CAD build for the part. Positions are in the model's coordinates, mm. Face numbers are marked on the shaded views. A direction names the side the tool comes from. Coordinates: 2 decimals unless noted, no trailing zeros. Loops run counter-clockwise (first coordinate to the right, second up) from the corner with the lowest first, then second, coordinate; pieces in that order, holes last. Notation, with made-up numbers: (-25, 1.25) - (30, 1.25) arc R21 ccw to (30, 22.25) - close; hole circle Ø3 at (-36.75, 60). An arc over 180 degrees is marked (long way). Put each result on its own line as item: value.
Autodesk Inventor part; units mm, degrees
ref_plane "YZ Plane" through (0, 0, 0) normal (1, 0, 0) x (0, 1, 0)
ref_plane "XZ Plane" through (0, 0, 0) normal (0, 1, 0) x (-1, 0, 0)
ref_plane "XY Plane" through (0, 0, 0) normal (0, 0, 1) x (1, 0, 0)
sketch "Sketch1" plane through (0, 0, 0) normal (0, 1, 0) x (-1, 0, 0)
  line L0 (150, 125) -> (-150, 125)
  line L1 (-150, 125) -> (-150, -125)
  line L2 (-150, -125) -> (150, -125)
  line L3 (150, -125) -> (150, 125)
  point P0 (0, 0)
  dimension "d0" = 300
  dimension "d1" = 250
  dimension "d2" = 125
  dimension "d29" = 150
extrude "Plate1" add sketch "Sketch1" along normal blind 9.5
sketch "Sketch4" plane through (0, 9.5, 0) normal (0, 1, 0) x (1, 0, 0)
  line L0 (-106, -70) -> (106, -70)
  line L1 (106, -70) -> (106, 70)
  line L2 (106, 70) -> (-106, 70)
  line L3 (-106, 70) -> (-106, -70)
  line L4 (-150, -125) -> (-150, 125)
  point P0 (0, 0)
  point P1 (-130, -106)
  point P2 (-130, 106)
  dimension "d24" = 140
  dimension "d25" = 212
  dimension "d27" = 70
  dimension "d28" = 106
hole "Hole1" at (-106, 9.5, 70) at (-106, 9.5, -70) at (106, 9.5, 70) at (106, 9.5, -70) direction (0, -1, 0) diameter 12 depth 9.5
sketch "Sketch8" plane through (-140.5, 9.5, 125) normal (-1, 0, 0) x (0, 1, 0)
  line L0 (0, -250) -> (0, 0)
  line L1 (0, 0) -> (-64.5, 0)
  line L2 (-64.5, 0) -> (-64.5, -250)
  line L3 (-64.5, -250) -> (0, -250)
edge flange "Flange5" height 64.5 angle 90 thickness 9.5 bend radius 9.5 thickness toward (-1, 0, 0) relief tear relief width 9.5 relief depth 4.75 edges at (-150, 9.5, 0) wall of the first edge with corners at (-140.5, 9.5, -125) (-140.5, 9.5, 125) (-140.5, -55, 125) (-140.5, -55, -125)
bend "Bend5"
corner "Corner5"
sketch "Sketch9" plane through (140.5, 9.5, -125) normal (1, 0, 0) x (0, -1, 0)
  line L0 (0, 250) -> (0, 0)
  line L1 (0, 0) -> (64.5, 0)
  line L2 (64.5, 0) -> (64.5, 250)
  line L3 (64.5, 250) -> (0, 250)
edge flange "Flange6" height 64.5 angle 90 thickness 9.5 bend radius 9.5 thickness toward (1, 0, 0) relief tear relief width 9.5 relief depth 4.75 edges at (150, 9.5, 0) wall of the first edge with corners at (140.5, 9.5, 125) (140.5, 9.5, -125) (140.5, -55, -125) (140.5, -55, 125)
bend "Bend6"
corner "Corner6"
sketch "Sketch10" plane through (-140.5, -45.5, -125) normal (0, -1, 0) x (-1, 0, 0)
  line L0 (0, 250) -> (0, 0)
  line L1 (0, 0) -> (54.5, 0)
  line L2 (54.5, 0) -> (54.5, 250)
  line L3 (54.5, 250) -> (0, 250)
edge flange "Flange7" height 45 angle 90 thickness 9.5 bend radius 9.5 thickness toward (0, -1, 0) relief tear relief width 9.5 relief depth 4.75 edges at (-140.5, -55, 0) wall of the first edge with corners at (-140.5, -45.5, 125) (-140.5, -45.5, -125) (-195, -45.5, -125) (-195, -45.5, 125)
bend "Bend7"
corner "Corner7"
sketch "Sketch11" plane through (140.5, -45.5, 125) normal (0, -1, 0) x (-1, 0, 0)
  line L0 (0, -250) -> (0, 0)
  line L1 (0, 0) -> (-54.5, 0)
  line L2 (-54.5, 0) -> (-54.5, -250)
  line L3 (-54.5, -250) -> (0, -250)
edge flange "Flange8" height 45 angle 90 thickness 9.5 bend radius 9.5 thickness toward (0, -1, 0) relief tear relief width 9.5 relief depth 4.75 edges at (140.5, -55, 0) wall of the first edge with corners at (140.5, -45.5, -125) (140.5, -45.5, 125) (195, -45.5, 125) (195, -45.5, -125)
bend "Bend8"
corner "Corner8"
sketch "Sketch12" plane through (-195, -45.5, 125) normal (0, 1, 0) x (1, 0, 0)
  line L0 (35.5, 250) -> (0, 250)
  line L1 (17.75, 250) -> (17.75, 0)
  line L2 (35.5, 0) -> (0, 0)
  line L3 (0, 0) -> (0, 250)
  line L4 (0, 195) -> (35.5, 195)
  line L5 (0, 55) -> (35.5, 55)
  line L6 (35.5, 250) -> (35.5, 0)
  point P0 (195, 125)
  point P1 (17.75, 195)
  point P2 (17.75, 55)
  dimension "d110" = 55
  dimension "d111" = 55
hole "Hole3" at (-177.25, -45.5, -70) at (-177.25, -45.5, 70) direction (0, -1, 0) diameter 12 depth 9.5
mirror "Mirror2" about plane through (0, 0, 0) normal (1, 0, 0) of "Hole3"
equation "\"d35\" = Thickness"
equation "\"d117\" = Thickness"
equation "\"d3\" = Thickness"
equation "\"d69\" = BendReliefWidth"
equation "\"d70\" = BendReliefDepth"
equation "\"d71\" = MinimumRemnant"
equation "\"d72\" = TransitionRadius"
equation "\"d75\" = BendRadius"
equation "\"d76\" = CornerReliefSize"
equation "\"d77\" = GapSize"
equation "\"d78\" = JacobiRadiusSize"
equation "\"d79\" = BendReliefWidth"
equation "\"d80\" = BendReliefDepth"
equation "\"d81\" = MinimumRemnant"
equation "\"d82\" = TransitionRadius"
equation "\"d85\" = BendRadius"
equation "\"d86\" = CornerReliefSize"
equation "\"d87\" = GapSize"
equation "\"d88\" = JacobiRadiusSize"
equation "\"d89\" = BendReliefWidth"
equation "\"d90\" = BendReliefDepth"
equation "\"d91\" = MinimumRemnant"
equation "\"d92\" = TransitionRadius"
equation "\"d95\" = BendRadius"
equation "\"d96\" = CornerReliefSize"
equation "\"d97\" = GapSize"
equation "\"d98\" = JacobiRadiusSize"
equation "\"d99\" = BendReliefWidth"
equation "\"d100\" = BendReliefDepth"
equation "\"d101\" = MinimumRemnant"
equation "\"d102\" = TransitionRadius"
equation "\"d105\" = BendRadius"
equation "\"d106\" = CornerReliefSize"
equation "\"d107\" = GapSize"
equation "\"d108\" = JacobiRadiusSize"
equation "\"BendRadius\" = Thickness"
equation "\"BendReliefWidth\" = Thickness"
equation "\"BendReliefDepth\" = 0.5 * Thickness"
equation "\"CornerReliefSize\" = 4 * Thickness"
equation "\"MinimumRemnant\" = 2 * Thickness"
equation "\"TransitionRadius\" = BendRadius"
equation "\"JacobiRadiusSize\" = BendRadius"
equation "\"GapSize\" = Thickness"
properties part number "BaseMotor" material "Steel ASTM A36"
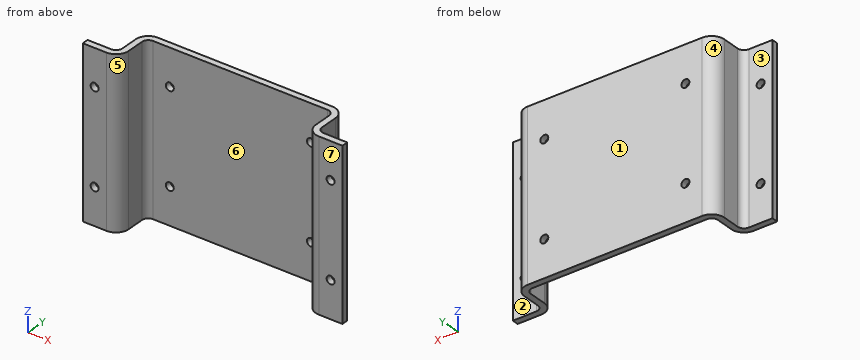
Q1. Mould opens along X. For the marked faces 4, 5, 6 and 7 say: +X half, -X half, draft (parallel to the pull), parting line (faces both ways), or undercut.
Determined:
face 4: -X half
face 5: undercut
face 6: undercut
face 7: draft
Q2. Pin check, flat tips, straight feed: pin 1 Ø10.5 at (x, z) = (-185.5, -53.5) entering from +Y; pin 2 Ø8 at (y, z) = (-23, 0.5) entering from -X; pin 3 Ø11 at (x, z) = (106, 70) entering from -Y; pin 4 Ø14 at (x, z) = (-106, -70) entering from +Y. Stop position of each tip, or through.
Determined:
pin 1: y = -45.5
pin 2: x = -150
pin 3: through
pin 4: y = 9.5
Q3. Slice it at D-D, the plane x = -118.5. Give the cut face in (y, z).
Determined:
outline: (0, -125) - (9.5, -125) - (9.5, 125) - (0, 125) - close
Q4. Slice it at B-B, the plane z = -37.5. Give the cut face in (x, y).
Determined:
outline: (-195, -55) - (-159.5, -55) arc R19 ccw to (-140.5, -36) - (-140.5, -9.5) arc R9.5 cw to (-131, 0) - (131, 0) arc R9.5 cw to (140.5, -9.5) - (140.5, -36) arc R19 ccw to (159.5, -55) - (195, -55) - (195, -45.5) - (159.5, -45.5) arc R9.5 cw to (150, -36) - (150, -9.5) arc R19 ccw to (131, 9.5) - (-131, 9.5) arc R19 ccw to (-150, -9.5) - (-150, -36) arc R9.5 cw to (-159.5, -45.5) - (-195, -45.5) - close
Q5. Tool access for the marked faces 1, 2 and 3: list every direction of +Z, -Z, +X, -X, +Y, -Y with a clear straight run to the whole face (end or side of a thin tool).
Determined:
face 1: +Z, -Z, +X, -X, +Y
face 2: +Z, -Z, +X, +Y
face 3: +Z, -Z, -X, +Y
Q6. Wall check: L1, parallel to Z at x = -177, y = -49; L2, parallel to X at y = -52.5, z = 70; L3, parallel to X at y = 7, z = -70. Give the ranges that are in metal, low to high. Write a range as from..to.
Determined:
L1: -125..-75.99, -64.01..64.01, 75.99..125
L2: -195..-183.25, -171.25..-150.08, 150.08..171.25, 183.25..195
L3: -140.42..-112, -100..100, 112..140.42
Q7. Slice it at C-C, the plane z = -70. State how many separate pieces and enclosed holes the cut face has, then the cut area to 3 significant figures.
Determined:
separate pieces: 5
enclosed holes: 0
area: 4,060 mm2
Q8. Slice it at A-A, the plane x = 106. Give the cut face in (y, z), then the cut area to 3 significant figures.
Determined:
outline: (0, -125) - (9.5, -125) - (9.5, -76) - (0, -76) - close; (0, -64) - (9.5, -64) - (9.5, 64) - (0, 64) - close; (0, 76) - (9.5, 76) - (9.5, 125) - (0, 125) - close
area: 2,150 mm2
